```python
from build123d import *

# Parameters (mm, degrees)
F0_W     = 40
F0_H     = 20
F1_DEPTH = 10
F2_W     = 40
F2_H     = 10
F3_DEPTH = 7
F5_D     = 3
F7_D     = 2


with BuildPart() as f1:
    # F0 (on Top) → F1 (new body)
    with BuildSketch(Plane.XY):
        Rectangle(F0_W, F0_H)
    extrude(amount=F1_DEPTH)

    # F2 (on face) → F3 (cut)
    with BuildSketch(Plane.XY.offset(10)):
        with Locations((0, 5)):
            Rectangle(F2_W, F2_H)
    extrude(amount=-F3_DEPTH, mode=Mode.SUBTRACT)

    # F5 (through all)
    with Locations(Plane.XZ.offset(10)):
        with Locations((0, 6)):
            Hole(F5_D / 2)

    # F7 (through all)
    with Locations(Plane.XY.offset(3)):
        with Locations((0, 5)):
            Hole(F7_D / 2)


solid = f1.part
```
Design review of the part built by this model. Coordinates are the model's own, in mm. A direction names the side the tool comes from. Coordinates: 2 decimals unless noted, no trailing zeros. Write each loop counter-clockwise with the first axis right and the second up, starting at its lowest first coordinate (ties: lowest second). Pieces come first, ordered by that corner, then holes.
1) Insertion check: pin 1 (4 mm diameter, centred on x = 0, z = 6, fed in from +Y); pin 2 (5 mm diameter, centred on x = 6.5, y = 7, fed in from +Z). Each pin has a flat end and moves straight along its axis. Give the tip position at first contact, or say it passes through.
2) Machinability: for faces 1 (the flat face through (0, 0, 8)), 2 (the flat face through (20, -2, 4)), which of the approach directions +Z, -Z, +X, -X, +Y, -Y give a long, thin tool a straight path to every point of the face, cutting with its end or side? Answer none if there is none.
3) Add section D-D (y = -1.25). Write out the cut boundary in (x, z), plus the area to 3 significant figures.
4) Mouldability with a two-part tool opening along Z and no side actions: class faces 3 (the flat face through (0, 0, 0)), 4 (the flat face through (0, -5, 10)), 5 (the cylindrical face through (0.325, -4.93, 4.536)), 6 (the flat face through (0, -10, 4)) as +Z half, -Z half, draft (parallel to the pull), parting line (faces both ways), or undercut.
5) Add section A-A (z = 6). Write out the cut boundary in (x, y), plus the area to 3 significant figures.
6) Add section B-B (y = 5). Write out the cut boundary in (x, z).
7) To check wall thickness, follow L1, parallel to Z at x = 0, y = -7; L2, parallel to Y at x = 0, z = 2.2; L3, parallel to Z at x = 2.5, y = 1.25. State the ranges of each line that lie inside material, in increasing order.
8) Add section C-C (x = 0). Write out the cut boundary in (y, z), plus the area to 3 significant figures.
Check result:
1. pin 1: stops at y = 0
1. pin 2: stops at z = 3
2. face 1: +Z, +X, -X, +Y
2. face 2: +Z, -Z, +X, +Y, -Y
3. outline: (-20, 0) - (20, 0) - (20, 10) - (-20, 10) - close; hole circle Ø3 at (0, 6)
3. area: 393 mm2
4. face 3: -Z half
4. face 4: +Z half
4. face 5: undercut
4. face 6: draft
5. outline: (-20, -10) - (-1.5, -10) - (-1.5, 0) - (-20, 0) - close; (1.5, -10) - (20, -10) - (20, 0) - (1.5, 0) - close
5. area: 370 mm2
6. outline: (-20, 0) - (-1, 0) - (-1, 3) - (-20, 3) - close; (1, 0) - (20, 0) - (20, 3) - (1, 3) - close
7. L1: z = 0 to 4.5, 7.5 to 10
7. L2: y = -10 to 4, 6 to 10
7. L3: z = 0 to 3
8. outline: (-10, 0) - (4, 0) - (4, 3) - (0, 3) - (0, 4.5) - (-10, 4.5) - close; (-10, 7.5) - (0, 7.5) - (0, 10) - (-10, 10) - close; (6, 0) - (10, 0) - (10, 3) - (6, 3) - close
8. area: 94.0 mm2
